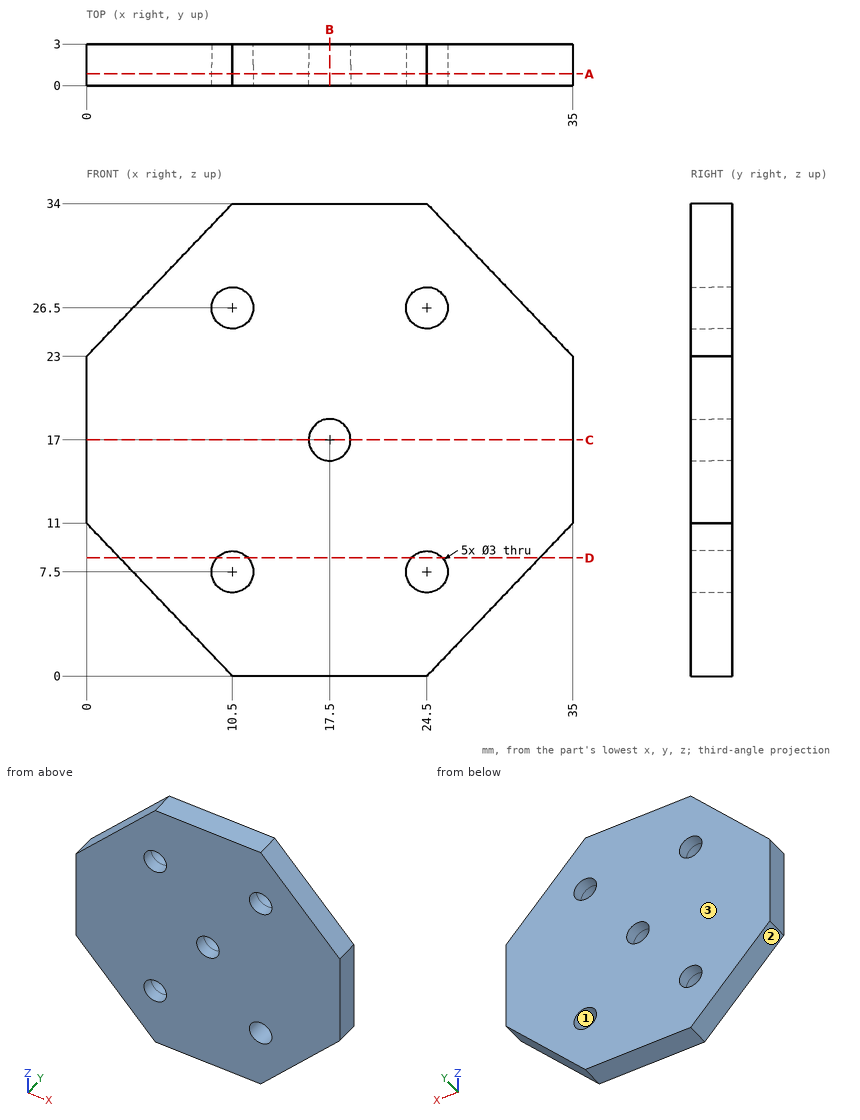
Could you check a few things on this drawing? It's one solid part, dimensions in mm from its lowest x, y, z. Give positions to 0.01 mm unless a question says otherwise; leave off trailing zeros. Order: outer loops, then holes, each group sorted by start corner. A loop starts at its lowest first (then second) coordinate and runs counter-clockwise, first axis right, second up. Notation, with made-up numbers: (2.25, -25) - (31.25, -25) arc R12 ccw to (31.25, -11) - close; hole circle Ø5 at (55, 79.5). An arc over 180 degrees is marked (long way). One line per item, written item: value. Start each with the question number.
1. If I drill on probe 1 along Z at (x, y) = (10.5, 2.05); probe 2 along Z at (x, y) = (11, 2); probe 3 along Z at (x, y) = (17.5, 2.1), over which ranges is the centre line in solid material (lowest first)?
2. Thinking about a two-plate mould opening in Z: for the marked faces 1, 2 and 3, which applies, +Z half, -Z half, draft (parallel to the pull), parting line (faces both ways), or undercut?
3. Imagine slicing it at C-C on z = 17. List the corners of the cut face in (x, y) for me, plus the area to 3 significant figures.
4. For P1, Ø2.5, axis at x = 24.5, z = 26.5, coming from the +Y side, with a flat end and sliding along its axis, tell me the tip position at first contact or that it passes through.
5. Imagine slicing it at A-A on y = 0.85. List the corners of the cut face in (x, z) for me, plus the area to 3 significant figures.
6. Imagine slicing it at D-D on z = 8.5. List the corners of the cut face in (x, y) for me.
7. Imagine slicing it at B-B on x = 17.5. List the corners of the cut face in (y, z) for me, plus the area to 3 significant figures.
Values:
1. probe 1: 0 to 6, 9 to 25, 28 to 34
1. probe 2: 0 to 6.09, 8.91 to 25.09, 27.91 to 34
1. probe 3: 0 to 15.5, 18.5 to 34
2. face 1: undercut
2. face 2: -Z half
2. face 3: draft
3. outline: (0, 0) - (16, 0) - (16, 3) - (0, 3) - close; (19, 0) - (35, 0) - (35, 3) - (19, 3) - close
3. area: 96.0 mm²
4. P1: through
5. outline: (0, 11) - (10.5, 0) - (24.5, 0) - (35, 11) - (35, 23) - (24.5, 34) - (10.5, 34) - (0, 23) - close; hole circle Ø3 at (10.5, 7.5); hole circle Ø3 at (10.5, 26.5); hole circle Ø3 at (17.5, 17); hole circle Ø3 at (24.5, 7.5); hole circle Ø3 at (24.5, 26.5)
5. area: 924 mm²
6. outline: (2.39, 0) - (9.38, 0) - (9.38, 3) - (2.39, 3) - close; (11.62, 0) - (23.38, 0) - (23.38, 3) - (11.62, 3) - close; (25.62, 0) - (32.61, 0) - (32.61, 3) - (25.62, 3) - close
7. outline: (0, 0) - (3, 0) - (3, 15.5) - (0, 15.5) - close; (0, 18.5) - (3, 18.5) - (3, 34) - (0, 34) - close
7. area: 93.0 mm²
